Geometry check sheet. Reference: the model listing, model coordinates, mm. Round coordinates to 2 decimals unless told otherwise and drop trailing zeros. Order: outer loops, then holes, each group sorted by start corner. A loop starts at its lowest first (then second) coordinate and runs counter-clockwise, first axis right, second up. Notation, with made-up numbers: (38.25, -38) - (44.25, -38) arc R19 cw to (44.25, -3) - close; hole circle Ø1 at (-35.5, 17.5). An arc over 180 degrees is marked (long way). Return JSON: item names as keys, results as strings. Group by question number.
Q1. Gauge pin test, flat ends, axial feed: pin 1 Ø10 at (x, z) = (336.55, 0) entering from -Y (3 decimals); pin 2 Ø2 at (x, y) = (82, 3) entering from +Z; pin 3 Ø8 at (x, y) = (157.5, -7.5) entering from +Z; pin 4 Ø1.5 at (x, y) = (224.5, -6.5) entering from +Z. Record the tip position at first contact, or that the pin passes through.
Q2. Sectioned sample at C-C, the plane x = 19.05. Record the cut outline in (y, z) (3 decimals), then the cut area to 3 significant figures.
Q3. Sectioned sample at D-D, the plane x = 176. Record the cut outline in (y, z) (3 decimals), then the cut area to 3 significant figures.
Q4. Draft check along Z on faces 1 (the cylindrical face through (175.311, 9.085, 2.861)), 2 (the flat face through (0, -2, 8)), 3 (the cylindrical face through (21.98, 8.45, -1.22)). Enter one of: pulls with the +Z half, pulls with the -Z half, needs draft (parallel to the pull), parting line crosses it, or undercut.
Q5. Sectioned sample at A-A, the plane y = 0. Record the cut outline in (x, z) (3 decimals).
Q6. Material ranges on line 1 along X through (y, z) = (8.7, 0) (3 decimals); line 2 along Y through (x, z) = (15.5, 0) (3 decimals); line 3 along X through (y, z) = (-7.75, 2.75), recorded low to high.
Q7. Sectioned sample at B-B, the plane z = 0. Record the cut outline in (x, y) (3 decimals).
```python
from build123d import *

# Parameters (mm, degrees)
F0_R     = 9.525
F0_R_2   = 8.0518
F1_DEPTH = 355.6
F2_R     = 3.175
F3_DEPTH = 38.1


with BuildPart() as f1:
    # F0 (on Right) → F1 (new body)
    with BuildSketch(Plane.YZ):
        Circle(F0_R)
        Circle(F0_R_2, mode=Mode.SUBTRACT)
    extrude(amount=F1_DEPTH)

    # F2 (on Front) → F3 (cut, symmetric)
    with BuildSketch(Plane.XZ):
        with Locations((336.55, 0)):
            Circle(F2_R)
        with Locations((19.05, 0)):
            Circle(F2_R)
    extrude(amount=F3_DEPTH, both=True, mode=Mode.SUBTRACT)


solid = f1.part
```
Reply:
{
 "1": {"pin 1": "y = -9.525", "pin 2": "z = 9.31", "pin 3": "z = 8.86", "pin 4": "z = 7.59"},
 "2": {"outline": "(-8.98, -3.175) arc R9.525 ccw to (8.98, -3.175) - (7.399, -3.175) arc R8.052 cw to (-7.399, -3.175) - close; (-8.98, 3.175) - (-7.399, 3.175) arc R8.052 cw to (7.399, 3.175) - (8.98, 3.175) arc R9.525 ccw to start", "area": "62.2 mm^2"},
 "3": {"outline": "circle Ø19.05 at (0, 0); hole circle Ø16.104 at (0, 0)", "area": "81.3 mm^2"},
 "4": {"face 1": "parting line crosses it", "face 2": "needs draft", "face 3": "undercut"},
 "5": {"outline": "(0, -9.525) - (355.6, -9.525) - (355.6, -8.052) - (0, -8.052) - close; (0, 8.052) - (355.6, 8.052) - (355.6, 9.525) - (0, 9.525) - close"},
 "6": {"line 1": "0 to 15.875, 22.225 to 333.375, 339.725 to 355.6", "line 2": "-9.525 to -8.052, 8.052 to 9.525", "line 3": "0 to 17.46, 20.64 to 334.96, 338.14 to 355.6"},
 "7": {"outline": "(0, -9.525) - (15.875, -9.525) - (15.875, -8.052) - (0, -8.052) - close; (0, 8.052) - (15.875, 8.052) - (15.875, 9.525) - (0, 9.525) - close; (22.225, -9.525) - (333.375, -9.525) - (333.375, -8.052) - (22.225, -8.052) - close; (22.225, 8.052) - (333.375, 8.052) - (333.375, 9.525) - (22.225, 9.525) - close; (339.725, -9.525) - (355.6, -9.525) - (355.6, -8.052) - (339.725, -8.052) - close; (339.725, 8.052) - (355.6, 8.052) - (355.6, 9.525) - (339.725, 9.525) - close"}
}
